Verification items for this drawing (mm, ordinates from the low corner). Give positions to 0.01 mm unless a question says otherwise; leave off trailing zeros. Loops run counter-clockwise (first coordinate to the right, second up) from the corner with the lowest first, then second, coordinate; pieces in that order, holes last. Notation, with made-up numbers: M -39.75,52 L -12.75,52 A26 cw -12.75,77 Z; hole C 47.5,-9.75 d4. An arc over 180 degrees is marked long. Put each result on its own line as item: value. Start each with the question number.
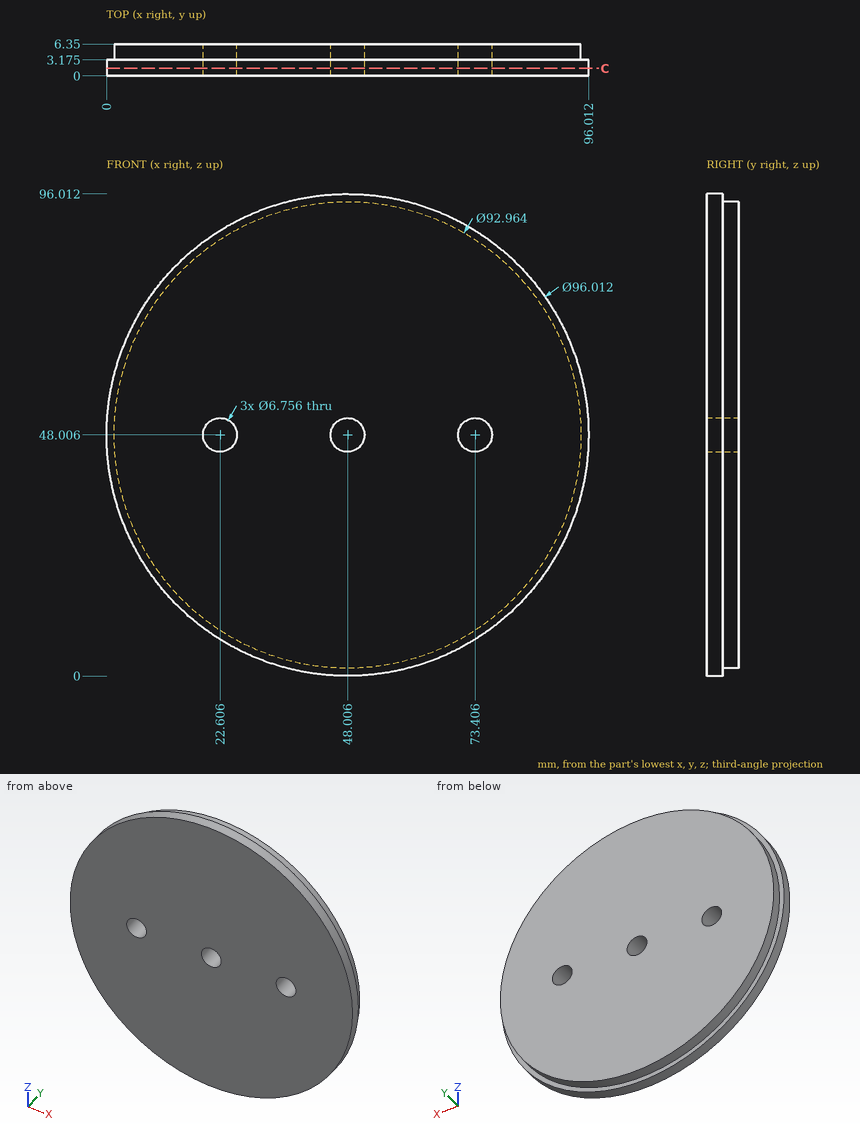
Q1. Scan lines: L1, parallel to X at y = 3, z = 49.5 (1 decimal); L2, parallel to Z at x = 22, y = 3 (1 decimal); L3, parallel to Z at x = 48.5, y = 2 (1 decimal). Record each from-to range of solid material in increasing order.
Q2. Go/stop test with flat-tipped pins: pin 1 (3 mm diameter, centred on x = 48, y = 4, fed in from +Z); pin 2 (6 mm diameter, centred on x = 56.5, z = 11, fed in from -Y); pin 3 (3 mm diameter, centred on x = 38, y = 4, fed in from +Z); pin 4 (2 mm diameter, centred on y = 2, z = 76.5, fed in from -X). Record where each tip stops, or that it passes through.
Q3. Cross-section at C-C, the plane y = 1.5. Record the boundary of the cut face in (x, z) (1 decimal).
Ans:
1. L1: x = 0 to 19.6, 25.6 to 45, 51 to 70.4, 76.4 to 96
1. L2: z = 7.7 to 44.7, 51.3 to 88.4
1. L3: z = 0 to 44.7, 51.3 to 96
2. pin 1: stops at z = 96.01
2. pin 2: stops at y = 0
2. pin 3: stops at z = 95.21
2. pin 4: stops at x = 8.65
3. outline: C 48,48 d96; hole C 22.6,48 d6.8; hole C 48,48 d6.8; hole C 73.4,48 d6.8
